Here's how the part is built. I have some questions about the finished solid (model axes, mm). Face numbers are marked on the shaded views. Round coordinates to 2 decimals unless told otherwise and drop trailing zeros. Write each loop counter-clockwise with the first axis right and the second up, starting at its lowest first coordinate (ties: lowest second). Pieces come first, ordered by that corner, then holes. Notation, with made-up numbers: (33.5, -29) - (43.5, -29) arc R32 cw to (43.5, 4) - close; hole circle Ø6 at (-29, 42.5). An arc over 180 degrees is marked (long way). One line per item, written item: value. Start each with the question number.
Item 1: Imagine slicing it at B-B, the plane x = 8.35. Please give me the cut outline in (y, z), then the cut area to 3 significant figures.
Item 2: Imagine slicing it at A-A, the plane y = 68. Please give me the cut outline in (x, z), then the cut area to 3 significant figures.
Item 3: Imagine slicing it at D-D, the plane x = 79.5. Please give me the cut outline in (y, z).
Item 4: If I drill on line 1 (Y direction, x = -8, z = 4.5); line 2 (X direction, y = 72.5, z = 62.4); line 3 (X direction, y = 12, z = 31.5), over which ranges is the centre line in solid material (lowest first)?
Item 5: For P1, Ø1.5, axis at y = 26.5, z = 62.5, coming from the -X side; P2, Ø2, axis at x = 18, z = 20, coming from the +Y side; P3, Ø4, axis at x = -8.35, y = 47.5, coming from the +Z side; P4, Ø5.5, axis at x = -97, y = 6, coming from the -Z side, each with a flat end and sliding along its axis, tell me the tip position at first contact or that it passes through.
Item 6: Thinking about a two-plate mould opening in Z: for the marked faces 1, 2 and 3, which applies, released by +Z, released by -Z, zero draft, split by the parting line, or undercut?
Item 7: Imagine slicing it at C-C, the plane z = 18. Please give me the cut outline in (x, y), then the cut area to 3 significant figures.
Autodesk Inventor part; units mm, degrees
ref_plane "Work Plane2" through (0, -2.5, 0) normal (-1, 0, 0) x (0, 0, 1)
ref_plane "Work Plane3" through (0, 0, 33) normal (0, 0, -1) x (-1, 0, 0)
ref_plane "YZ Plane" through (0, 0, 0) normal (1, 0, 0) x (0, 1, 0)
sketch "Sketch1" plane through (0, 0, 0) normal (0, 0, 1) x (1, 0, 0)
  line L0 (100, -2.5) -> (-100, -2.5)
  line L1 (-100, -2.5) -> (-100, 2.5)
  line L2 (-100, 2.5) -> (100, 2.5)
  line L3 (100, 2.5) -> (100, -2.5)
  line L4 (100, -2.5) -> (-100, 2.5) construction
  line L5 (-100, -2.5) -> (100, 2.5) construction
  point P0 (0, 0)
  dimension "d0" = 200
  dimension "d1" = 5
extrude "Extrusion1" add sketch "Sketch1" along normal blind 66
sketch "Sketch2" plane through (0, 0, 0) normal (0, 0, -1) x (-1, 0, 0)
  line L0 (-8.35, 72.5) -> (8.35, 72.5)
  line L1 (8.35, 72.5) -> (8.35, 47.5)
  line L2 (8.35, 47.5) -> (-8.35, 47.5)
  line L3 (-8.35, 47.5) -> (-8.35, 72.5)
  line L4 (-8.35, 72.5) -> (8.35, 47.5) construction
  line L5 (8.35, 72.5) -> (-8.35, 47.5) construction
  line L6 (-13.35, -2.5) -> (13.35, -2.5)
  line L7 (13.35, -2.5) -> (13.35, 77.5)
  line L8 (13.35, 77.5) -> (-13.35, 77.5)
  line L9 (-13.35, 77.5) -> (-13.35, -2.5)
  line L10 (-13.35, -2.5) -> (13.35, 77.5) construction
  line L11 (13.35, -2.5) -> (-13.35, 77.5) construction
  circle A0 centre (-8.35, 47.5) radius 2.5
  circle A1 centre (8.35, 47.5) radius 2.5
  circle A2 centre (8.35, 72.5) radius 2.5
  circle A3 centre (-8.35, 72.5) radius 2.5
  line L12 (-100, 2.5) -> (100, 2.5)
  line L13 (100, -2.5) -> (-100, -2.5)
  point P0 (0, -2.5)
  dimension "d4" = 25
  dimension "d5" = 16.7
  dimension "d6" = 5
  dimension "d7" = 5
  dimension "d8" = 5
  dimension "d11" = 5
  dimension "d12" = 5
  dimension "d13" = 5
  dimension "d14" = 5
  dimension "d33" = 50
extrude "Extrusion3" cut sketch "Sketch2" along normal blind 5 contours L3 A3 L0 | L0 A3 L3 | A2 L1 L0 | L0 L1 A2 | A0 L2 L3 | L3 L2 A0 | A1 L2 L1 | L1 L2 A1
sketch "Sketch3" plane through (-100, 2.5, 66) normal (0, 1, 0) x (1, 0, 0)
  line L0 (200, 66) -> (0, 66)
  line L1 (0, 66) -> (0, 0)
  line L2 (200, 0) -> (0, 0)
  line L3 (200, 66) -> (200, 0)
  line L4 (0, 66) -> (0, 0)
  line L5 (200, 66) -> (200, 0)
  line L6 (100, 33) -> (100, 66)
  line L7 (100, 33) -> (100, 0)
  line L8 (0, 0) -> (200, 0)
  line L9 (100, 33) -> (200, 33)
  circle A0 centre (100, 33) radius 4
  circle A1 centre (150, 33) radius 4
  line L10 (100, 33) -> (200, 33)
  line L11 (200, 66) -> (200, 0)
  line L12 (150, 33) -> (100, 33)
  dimension "d17" = 8
  dimension "d18" = 8
  dimension "d23" = 50
sketch "Sketch5" plane through (-100, -2.5, 0) normal (-1, 0, 0) x (0, 0, 1)
  circle A0 centre (33, 10) radius 2.5
  circle A1 centre (33, 10) radius 5
  line L0 (0, 5) -> (0, 20)
  line L1 (0, 5) -> (66, 5)
  line L2 (0, 5) -> (66, 5)
  line L3 (28, 5) -> (28, 10)
  line L4 (38, 5) -> (38, 10)
  point P0 (0, 2.5)
  point P1 (33, 5)
  point P2 (28, 5)
  point P3 (38, 5)
  dimension "d29" = 5
  dimension "d30" = 10
extrude "Extrusion7" add sketch "Sketch5" against normal blind 10
ref_plane "Work Plane2" through (0, -2.5, 0) normal (-1, 0, 0) x (0, 0, 1)
mirror "Mirror2" about plane through (0, -2.5, 0) normal (-1, 0, 0) of "Extrusion7"
extrude "Extrusion8" add sketch "Sketch2" against normal blind 5 contours L0 A2 L1 A1 L2 A0 L3 A3 | L9 L12 L7 L6 | L9 L8 L7 L12
ref_plane "Work Plane3" through (0, 0, 33) normal (0, 0, -1) x (-1, 0, 0)
mirror "Mirror3" about plane through (0, 0, 33) normal (0, 0, -1) of "Extrusion8"
properties part number "FP V2 Mounting Plate" material "Aluminum 6061"
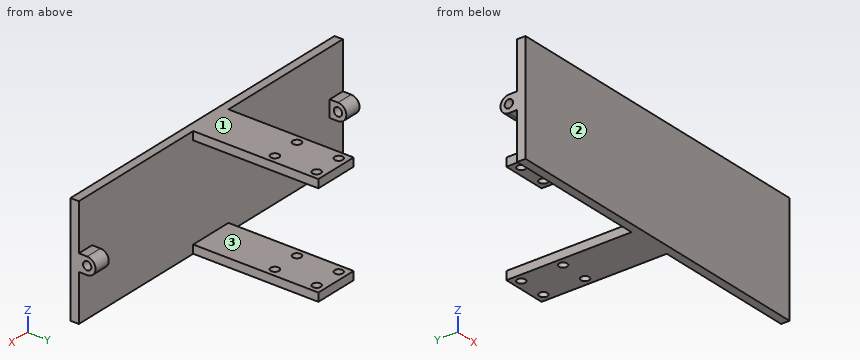
Values follow:
1. outline: (-2.5, 0) - (45, 0) - (45, 5) - (2.5, 5) - (2.5, 61) - (45, 61) - (45, 66) - (-2.5, 66) - close; (50, 0) - (70, 0) - (70, 5) - (50, 5) - close; (50, 61) - (70, 61) - (70, 66) - (50, 66) - close; (75, 0) - (77.5, 0) - (77.5, 5) - (75, 5) - close; (75, 61) - (77.5, 61) - (77.5, 66) - (75, 66) - close
1. area: 980 mm^2
2. outline: (-13.35, 0) - (13.35, 0) - (13.35, 5) - (-13.35, 5) - close; (-13.35, 61) - (13.35, 61) - (13.35, 66) - (-13.35, 66) - close
2. area: 267 mm^2
3. outline: (-2.5, 0) - (2.5, 0) - (2.5, 66) - (-2.5, 66) - close
4. line 1: y = -2.5 to 45.02, 49.98 to 70.02, 74.98 to 77.5
4. line 2: x = -13.35 to -10.85, -5.85 to 5.85, 10.85 to 13.35
4. line 3: x = -100 to -90, 90 to 100
5. P1: stops at x = -13.35
5. P2: stops at y = 2.5
5. P3: passes through
5. P4: stops at z = 28
6. face 1: released by +Z
6. face 2: zero draft
6. face 3: undercut
7. outline: (-100, -2.5) - (100, -2.5) - (100, 2.5) - (-100, 2.5) - close
7. area: 1,000 mm^2
